For this review, take the finished solid that the model builds, in its own axes (mm). A direction names the side the tool comes from. Give positions to 0.01 mm unless a question says otherwise; leave off trailing zeros. Order: outer loops, then holes, each group sorted by start corner. A loop starts at its lowest first (then second) coordinate and runs counter-clockwise, first axis right, second up. Notation, with made-up numbers: M 74.5,44 L 123.5,44 A4 cw 123.5,48 Z; hole C 2.25,10.25 d10. An arc over 180 degrees is marked long. Answer as CSV lines item,"result". Start each with the question number.
1. We need section D-D, the plane y = -4.5. Give the boundary of the cut face in (x, z) (3 decimals).
2. Mouldability with a two-part tool opening along Y and no side actions: class faces 3 (the cylindrical face through (-45.814, -10.79, 0.966)), 4 (the flat face through (-1, 12.7, 1)), 5 (the cylindrical face through (34.93, 0.14, 0.94)) as pulls with the +Y half, pulls with the -Y half, needs draft (parallel to the pull), parting line crosses it, or undercut.
3. We need section B-B, the plane z = 0.9. Give the boundary of the cut face in (x, y) (3 decimals), and give its area (3 significant figures).
4. We need section C-C, the plane y = 0. Give the boundary of the cut face in (x, z) (3 decimals).
5. Clearance check with a flat-ended pin moving along its axis: P1, Ø7.5, axis at x = -38.1, y = 0, coming from the -Z side. State where the tip first meets the part, or that it passes through.
6. We need section A-A, the plane x = -38.1. Give the boundary of the cut face in (y, z) (3 decimals), and give its area (3 significant figures).
7. For line 1 along X through (y, z) = (2.25, 1.4) (3 decimals); line 2 along Y through (x, z) = (22, 0.35); line 3 along Y through (x, z) = (38.1, 1.2) (3 decimals), list the stretches that pass through material, from the lowest coordinate up.
8. Machinability: for faces 1 (the flat face through (0, -6.35, 1)), 2 (the flat face through (-1, -12.7, 1)), which of the approach directions +Z, -Z, +X, -X, +Y, -Y give a long, thin tool a straight path to every point of the face, cutting with its end or side? Answer none if there is none.
from build123d import *

# Parameters (mm, degrees)
SKETCH1_W           = 95.25
SKETCH1_H           = 25.4
SKETCH1_R           = 3.175
BOSS_EXTRUDE1_DEPTH = 1.905
CUT_EXTRUDE1_DEPTH  = 2.905
FILLET1_R           = 6.35


with BuildPart() as part:
    # Sketch1 → Boss-Extrude1 (new body)
    with BuildSketch(Plane.XY):
        Rectangle(SKETCH1_W, SKETCH1_H)
        with Locations((-38.1, 0)):
            Circle(SKETCH1_R, mode=Mode.SUBTRACT)
        with Locations((38.1, 0)):
            Circle(SKETCH1_R, mode=Mode.SUBTRACT)
    extrude(amount=BOSS_EXTRUDE1_DEPTH)

    # Sketch2 → Cut-Extrude1 (cut, through all)
    with BuildSketch(Plane.XY.offset(1.905)):
        with BuildLine():
            Line((-22.225, 6.35), (22.225, 6.35))
            ThreePointArc((22.225, 6.35), (28.575, 0), (22.225, -6.35))
            Line((22.225, -6.35), (-22.225, -6.35))
            ThreePointArc((-22.225, -6.35), (-28.575, 0), (-22.225, 6.35))
        make_face()
    extrude(amount=-CUT_EXTRUDE1_DEPTH, mode=Mode.SUBTRACT)

    # Fillet1
    fillet1_edges = [part.edges().sort_by_distance(p)[0] for p in [
        (47.625, -12.7, 0.9525),
        (-47.625, -12.7, 0.9525),
        (-47.625, 12.7, 0.9525),
        (47.625, 12.7, 0.9525),
    ]]
    fillet(fillet1_edges, radius=FILLET1_R)


solid = part.part
Result set:
1,outline,"M -47.625,0 L -26.705,0 L -26.705,1.905 L -47.625,1.905 Z; M 26.705,0 L 47.625,0 L 47.625,1.905 L 26.705,1.905 Z"
2,face 3,"pulls with the -Y half"
2,face 4,"pulls with the +Y half"
2,face 5,"undercut"
3,outline,"M -47.625,-6.35 A6.35 ccw -41.275,-12.7 L 41.275,-12.7 A6.35 ccw 47.625,-6.35 L 47.625,6.35 A6.35 ccw 41.275,12.7 L -41.275,12.7 A6.35 ccw -47.625,6.35 Z; hole C -38.1,0 d6.35; hole M -22.225,-6.35 L 22.225,-6.35 A6.35 ccw 22.225,6.35 L -22.225,6.35 A6.35 ccw Z; hole C 38.1,0 d6.35"
3,area,"1,630 mm2"
4,outline,"M -47.625,0 L -41.275,0 L -41.275,1.905 L -47.625,1.905 Z; M -34.925,0 L -28.575,0 L -28.575,1.905 L -34.925,1.905 Z; M 28.575,0 L 34.925,0 L 34.925,1.905 L 28.575,1.905 Z; M 41.275,0 L 47.625,0 L 47.625,1.905 L 41.275,1.905 Z"
5,P1,"z = 0"
6,outline,"M -12.7,0 L -3.175,0 L -3.175,1.905 L -12.7,1.905 Z; M 3.175,0 L 12.7,0 L 12.7,1.905 L 3.175,1.905 Z"
6,area,"36.3 mm2"
7,line 1,"-47.625 to -40.34, -35.86 to -28.163, 28.163 to 35.86, 40.34 to 47.625"
7,line 2,"-12.7 to -6.35, 6.35 to 12.7"
7,line 3,"-12.7 to -3.175, 3.175 to 12.7"
8,face 1,"+Z, -Z"
8,face 2,"+Z, -Z, +X, -X, -Y"
